Drawing for the job (mm, zero at the part's lowest x, y, z). Round coordinates to 2 decimals unless told otherwise and drop trailing zeros. Order: outer loops, then holes, each group sorted by start corner. A loop starts at its lowest first (then second) coordinate and runs counter-clockwise, first axis right, second up. Notation, with made-up numbers: (-16.5, -24.5) -> (25.5, -24.5) arc R18 ccw to (25.5, 0.5) -> close; hole circle Ø4 at (45.25, -2). An arc over 180 degrees is marked (long way). Use CSV: the item, a comma, the result in double quotes.
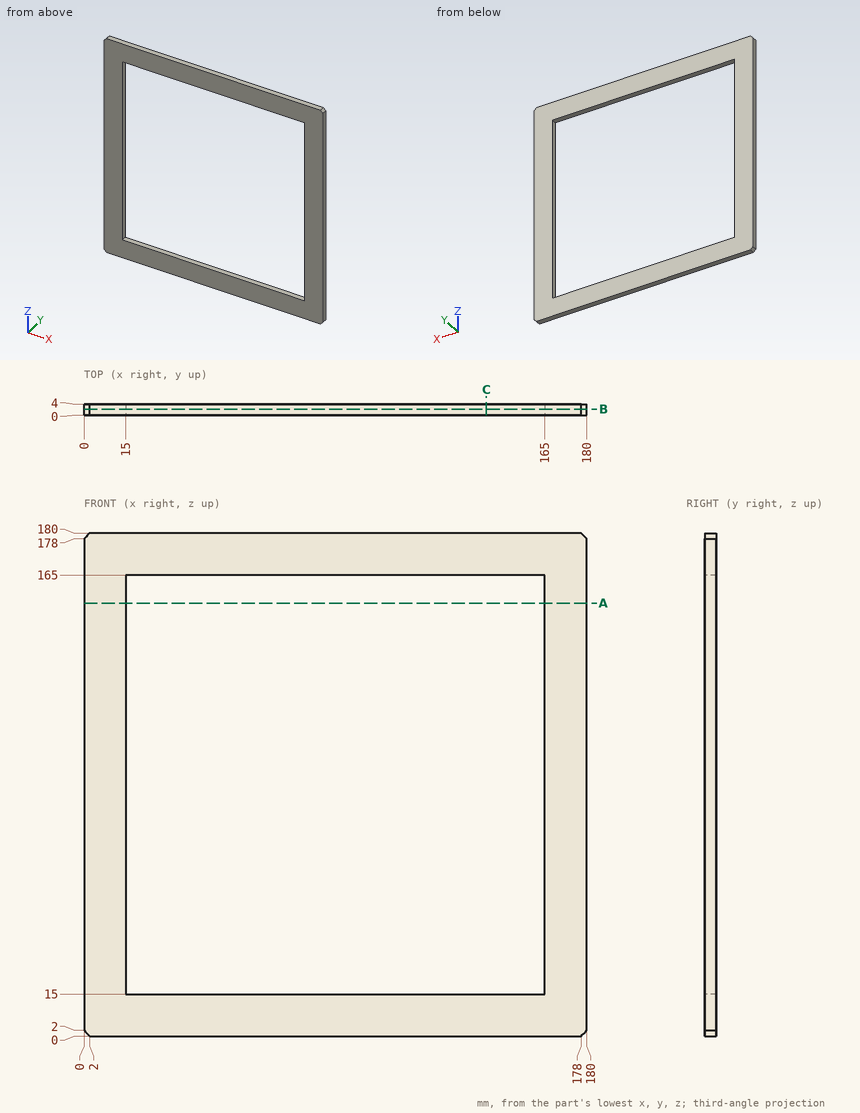
Q1. Cut at C-C (x = 144). Give the cut face in (y, z), plus the area to 3 significant figures.
From the geometry:
outline,"(0, 0) -> (4, 0) -> (4, 15) -> (0, 15) -> close; (0, 165) -> (4, 165) -> (4, 180) -> (0, 180) -> close"
area,"120 mm²"
Q2. Cut at B-B (y = 2.2). Give the cut face in (x, z).
From the geometry:
outline,"(0, 2) -> (2, 0) -> (178, 0) -> (180, 2) -> (180, 178) -> (178, 180) -> (2, 180) -> (0, 178) -> close; hole (15, 15) -> (165, 15) -> (165, 165) -> (15, 165) -> close"
Q3. Probe line 1 along Z through (x, y) = (23.5, 1.25). List the from-to ranges inside material, lowest first.
From the geometry:
line 1,"z = 0 to 15, 165 to 180"
Q4. Cut at A-A (z = 155). Give the cut face in (x, y).
From the geometry:
outline,"(0, 0) -> (15, 0) -> (15, 4) -> (0, 4) -> close; (165, 0) -> (180, 0) -> (180, 4) -> (165, 4) -> close"
